Verification items for the finished model (mm, model axes). A direction names the side the tool comes from. Give positions to 0.01 mm unless a question says otherwise; leave off trailing zeros. Loops run counter-clockwise (first coordinate to the right, second up) from the corner with the lowest first, then second, coordinate; pieces in that order, holes last. Notation, with made-up numbers: M 36.5,57.25 L 68.5,57.25 A21 ccw 68.5,79.25 Z; hole C -22.75,20 d5. An arc over 180 degrees is marked long. Use CSV: the item, a comma, the result in double quotes.
from build123d import *

# Parameters (mm, degrees)
SKETCH1_W           = 20
SKETCH1_H           = 15
SKETCH1_R           = 5
BOSS_EXTRUDE1_DEPTH = 20
SKETCH2_R           = 1.5
CUT_EXTRUDE2_DEPTH  = 20
SKETCH4_W           = 1.5
SKETCH4_H           = 7.5
SKETCH4_W_2         = 7.5
SKETCH4_H_2         = 1.5
BOSS_EXTRUDE3_DEPTH = 150
FILLET3_R           = 1


with BuildPart() as part:
    # Sketch1 → Boss-Extrude1 (new body)
    with BuildSketch(Plane(origin=(0, 0, 0), x_dir=(1, 0, 0), z_dir=(0, 1, 0))):
        Rectangle(SKETCH1_W, SKETCH1_H)
        Circle(SKETCH1_R, mode=Mode.SUBTRACT)
    extrude(amount=BOSS_EXTRUDE1_DEPTH)

    # Sketch2 → Cut-Extrude2 (cut)
    with BuildSketch(Plane.XY.offset(7.5)):
        with Locations((7.5, 10)):
            Circle(SKETCH2_R)
        with Locations((-7.5, 10)):
            Circle(SKETCH2_R)
    extrude(amount=-CUT_EXTRUDE2_DEPTH, mode=Mode.SUBTRACT)

    # Sketch4 → Boss-Extrude3 (add)
    with BuildSketch(Plane.XY.offset(7.5)):
        with Locations((0, 10)):
            Rectangle(SKETCH4_W, SKETCH4_H)
        with Locations((0, 10)):
            Rectangle(SKETCH4_W_2, SKETCH4_H_2)
    extrude(amount=BOSS_EXTRUDE3_DEPTH)

    # Fillet3
    fillet3_edges = [part.edges().sort_by_distance(p)[0] for p in [
        (-10, 20, 0),
        (10, 20, 0),
        (-10, 0, 0),
        (10, 0, 0),
    ]]
    fillet(fillet3_edges, radius=FILLET3_R)


solid = part.part
(1) Tool access check on faces 4 (the flat face through (0, 10, -7.5)), 5 (the flat face through (2, 9.25, 81)), 6 (the flat face through (-0.75, 12, 81)), 7 (the flat face through (-2, 9.25, 81)), 8 (the flat face through (0.75, 12, 81)). Record the directions out of +Z, -Z, +X, -X, +Y, -Y that give a thin tool (end or side, any length) a straight path to the whole face; none if there is none.
Calculated:
face 4,"-Z, +X, -X, +Y, -Y"
face 5,"+Z, +X, -Y"
face 6,"+Z, -X, +Y"
face 7,"+Z, -X, -Y"
face 8,"+Z, +X, +Y"
(2) Scan lines: L1, parallel to X at y = 10.25, z = 0; L2, parallel to X at y = 13.5, z = 0; L3, parallel to Y at x = 7.5, z = -4.25. Record each from-to range of solid material in increasing order. Write a range as from..to.
Calculated:
L1,"x = -10..-8.98, -6.02..-5, 5..6.02, 8.98..10"
L2,"x = -10..-5, 5..10"
L3,"y = 0..8.5, 11.5..20"
(3) Section check B-B on x = -7.5. Record the cut outline in (y, z).
Calculated:
outline,"M 0,-7.5 L 8.5,-7.5 L 8.5,7.5 L 0,7.5 Z; M 11.5,-7.5 L 20,-7.5 L 20,7.5 L 11.5,7.5 Z"
(4) Section check A-A on z = 0. Record the cut outline in (x, y).
Calculated:
outline,"M -10,1 A1 ccw -9,0 L -5,0 L -5,20 L -9,20 A1 ccw -10,19 Z; M 5,0 L 9,0 A1 ccw 10,1 L 10,19 A1 ccw 9,20 L 5,20 Z; hole C -7.5,10 d3; hole C 7.5,10 d3"
(5) Mould release check, pull along X, two halves, no side actions. Record for faces 1 (the cylindrical face through (6.3, 9.1, 0.1)), 2 (the flat face through (-10, 10, 0)), 3 (the flat face through (2, 10.75, 81)): released by +X, released by -X, zero draft, split by the parting line, or undercut.
Calculated:
face 1,"undercut"
face 2,"released by -X"
face 3,"zero draft"
(6) Section check C-C on z = 44.5. Record the cut outline in (x, y), plus the area to 4 significant figures.
Calculated:
outline,"M -3.75,9.25 L -0.75,9.25 L -0.75,6.25 L 0.75,6.25 L 0.75,9.25 L 3.75,9.25 L 3.75,10.75 L 0.75,10.75 L 0.75,13.75 L -0.75,13.75 L -0.75,10.75 L -3.75,10.75 Z"
area,"20.25 mm²"
(7) Depth check by flat-ended pin: pin 1 Ø3.5 at (x, y) = (7.5, 10) entering from +Z; pin 2 Ø10 at (x, y) = (3.5, 13) entering from +Z; pin 3 Ø3.5 at (x, z) = (-3, 68) entering from +Y; pin 4 Ø1.5 at (y, z) = (12.5, 82) entering from -X. Enter the tip coordinate at first touch or a pass-through.
Calculated:
pin 1,"stops at z = 7.5"
pin 2,"stops at z = 157.5"
pin 3,"stops at y = 10.75"
pin 4,"stops at x = -0.75"
